from build123d import *

# Parameters (mm, degrees)
SKETCH1_W           = 42.3
SKETCH1_H           = 49
SKETCH1_R           = 1.5
SKETCH1_R_2         = 11.5
BOSS_EXTRUDE1_DEPTH = 5
SKETCH2_W           = 42.3
SKETCH2_H           = 5
BOSS_EXTRUDE2_DEPTH = 42.3
SKETCH4_R           = 1.5
SKETCH4_R_2         = 13
CUT_EXTRUDE1_DEPTH  = 68.975087348
BOSS_EXTRUDE3_DEPTH = 3
BOSS_EXTRUDE4_DEPTH = 3
SKETCH8_R           = 3
CUT_EXTRUDE2_DEPTH  = 3
CUT_EXTRUDE3_DEPTH  = 72.905702138


with BuildPart() as part:
    # Sketch1 → Boss-Extrude1 (new body)
    with BuildSketch(Plane(origin=(0, 0, 0), x_dir=(1, 0, 0), z_dir=(0, 1, 0))):
        Rectangle(SKETCH1_W, SKETCH1_H)
        with Locations(Location((-15.5, 18.85, 0), (0, 0, 270))):
            Circle(SKETCH1_R, mode=Mode.SUBTRACT)
        with Locations(Location((15.5, 18.85, 0), (0, 0, 270))):
            Circle(SKETCH1_R, mode=Mode.SUBTRACT)
        with Locations(Location((-15.5, -12.15, 0), (0, 0, 90))):
            Circle(SKETCH1_R, mode=Mode.SUBTRACT)
        with Locations(Location((15.5, -12.15, 0), (0, 0, 90))):
            Circle(SKETCH1_R, mode=Mode.SUBTRACT)
        with Locations(Location((0, 3.35, 0), (0, 0, 270))):
            Circle(SKETCH1_R_2, mode=Mode.SUBTRACT)
    extrude(amount=BOSS_EXTRUDE1_DEPTH)

    # Sketch2 → Boss-Extrude2 (add)
    with BuildSketch(Plane(origin=(0, 5, 0), x_dir=(1, 0, 0), z_dir=(0, 1, 0))):
        with Locations((0, -22)):
            Rectangle(SKETCH2_W, SKETCH2_H)
    extrude(amount=BOSS_EXTRUDE2_DEPTH)

    # Sketch4 → Cut-Extrude1 (cut, through all)
    with BuildSketch(Plane(origin=(0, 0, 19.5), x_dir=(-1, 0, 0), z_dir=(0, 0, -1))):
        with Locations((-15, 41.15)):
            Circle(SKETCH4_R)
        with Locations((15, 41.15)):
            Circle(SKETCH4_R)
        with Locations(Location((-15, 11.15, 0), (0, 0, 180))):
            Circle(SKETCH4_R)
        with Locations(Location((15, 11.15, 0), (0, 0, 180))):
            Circle(SKETCH4_R)
        with Locations((0, 26.15)):
            Circle(SKETCH4_R_2)
    extrude(amount=-CUT_EXTRUDE1_DEPTH, mode=Mode.SUBTRACT)

    # Sketch5 → Boss-Extrude3 (add)
    with BuildSketch(Plane(origin=(21.15, 0, 0), x_dir=(0, 0, -1), z_dir=(1, 0, 0))):
        Polygon((-19.5, 47.3), (24.5, 5), (24.5, 0), (-24.5, 0), (-24.5, 47.3), align=None)
    extrude(amount=BOSS_EXTRUDE3_DEPTH)

    # Sketch6 → Boss-Extrude4 (add)
    with BuildSketch(Plane.ZY.offset(21.15)):
        Polygon((19.5, 47.3), (-24.5, 5), (-24.5, 0), (24.5, 0), (24.5, 47.3), align=None)
    extrude(amount=BOSS_EXTRUDE4_DEPTH)

    # Sketch8 → Cut-Extrude2 (cut)
    with BuildSketch(Plane(origin=(0, 0, 19.5), x_dir=(-1, 0, 0), z_dir=(0, 0, -1))):
        with Locations((-15, 41.15)):
            Circle(SKETCH8_R)
        with Locations((15, 41.15)):
            Circle(SKETCH8_R)
        with Locations((15, 11.15)):
            Circle(SKETCH8_R)
        with Locations((-15, 11.15)):
            Circle(SKETCH8_R)
    extrude(amount=-CUT_EXTRUDE2_DEPTH, mode=Mode.SUBTRACT)

    # Sketch9 → Cut-Extrude3 (cut, through all)
    with BuildSketch(Plane.ZY.offset(24.15)):
        Polygon((-12.084497186, 10), (14.5, 35.557368886), (14.5, 10), align=None)
    extrude(amount=-CUT_EXTRUDE3_DEPTH, mode=Mode.SUBTRACT)


solid = part.part
Could you check a few things on this model? Use its own coordinates, in mm. A direction names the side the tool comes from. Give positions to 0.01 mm unless a question says otherwise; leave off trailing zeros. Order: outer loops, then holes, each group sorted by start corner. A loop starts at its lowest first (then second) coordinate and runs counter-clockwise, first axis right, second up. Notation, with made-up numbers: (51.25, 43) -> (85.25, 43) arc R25 ccw to (85.25, 66) -> close; hole circle Ø6 at (-31, 84). An arc over 180 degrees is marked (long way). Answer in a Markdown table with one row per item. Add a question column.
Item 1: Imagine slicing it at A-A (y = 11.15). Count the separate pieces of the cut face and the enclosed holes in it, and give its area (3 significant figures).
Item 2: For faces 1 (the flat face through (-23, 10, 1)), 2 (the cylindrical face through (15.391, 44.124, 20.979)), 3 (the flat face through (-10, 16, 19.5)), which set-ups out of +Z, -Z, +X, -X, +Y, -Y let a thin tool reach every point of the face, with its end or its side?
Item 3: Imagine slicing it at B-B (x = 0). List the corners of the cut face in (y, z) for me, and give its area (4 significant figures).
Item 4: Imagine slicing it at C-C (z = -18.85). List the corners of the cut face in (x, y) for me, and give its area (3 significant figures).
Item 5: I'm going to push flat-ended pins straight in: P1, Ø5, axis at x = 12.5, z = -9.5, coming from the -Y side; P2, Ø3.5, axis at x = -15.5, z = -18.85, coming from the +Y side; P3, Ø3.5, axis at x = -15, y = 41.15, coming from the -Z side; P4, Ø1.5, axis at x = -23, z = -4.5, coming from the +Y side. Where does each tip first touch, or does it pass through?
Item 6: We'd pull the mould along Z, two halves only. Please class faces 4 (the cylindrical face through (15.95, 2.46, -17.42)), 5 (the flat face through (-16, 13, 22.5)), 6 (the flat face through (-21.15, 25, 1)): pulls with the +Z half, pulls with the -Z half, needs draft (parallel to the pull), parting line crosses it, or undercut.
Item 7: Please list where these lines run through material, in increasing order: probe 1 along Y at (x, z) = (-15, 24); probe 2 along X at (y, z) = (11.15, 23.6); probe 3 along X at (y, z) = (14, -11.5).
Result:
| question | item | result |
|---|---|---|
| 1 | separate pieces | 5 |
| 1 | enclosed holes | 0 |
| 1 | area | 267 mm2 |
| 2 | face 1 | +X, -X |
| 2 | face 2 | -Z |
| 2 | face 3 | -Z, +Y |
| 3 | outline | (0, -24.5) -> (5, -24.5) -> (5, -14.85) -> (0, -14.85) -> close; (0, 8.15) -> (5, 8.15) -> (5, 19.5) -> (13.15, 19.5) -> (13.15, 24.5) -> (0, 24.5) -> close; (39.15, 19.5) -> (47.3, 19.5) -> (47.3, 24.5) -> (39.15, 24.5) -> close |
| 3 | area | 211.5 mm2 |
| 4 | outline | (-24.15, 0) -> (-17, 0) -> (-17, 5) -> (-21.15, 5) -> (-21.15, 10.43) -> (-24.15, 10.43) -> close; (-14, 0) -> (14, 0) -> (14, 5) -> (-14, 5) -> close; (17, 0) -> (24.15, 0) -> (24.15, 10.43) -> (21.15, 10.43) -> (21.15, 5) -> (17, 5) -> close |
| 4 | area | 244 mm2 |
| 5 | P1 | y = 0 |
| 5 | P2 | y = 5 |
| 5 | P3 | z = 22.5 |
| 5 | P4 | y = 24.95 |
| 6 | face 4 | undercut |
| 6 | face 5 | pulls with the -Z half |
| 6 | face 6 | needs draft |
| 7 | probe 1 | 0 to 9.65, 12.65 to 39.65, 42.65 to 47.3 |
| 7 | probe 2 | -24.15 to -16.5, -13.5 to 13.5, 16.5 to 24.15 |
| 7 | probe 3 | -24.15 to -21.15, 21.15 to 24.15 |
